from build123d import *

# Parameters (mm, degrees)
SKETCH1_R           = 4.75
BOSS_EXTRUDE1_DEPTH = 9
SKETCH2_R           = 7.5
BOSS_EXTRUDE2_DEPTH = 200
CUT_EXTRUDE1_START  = 4
SKETCH3_W           = 10
SKETCH3_H           = 10
CUT_EXTRUDE1_DEPTH  = 206.268965688
CIRPATTERN2_COUNT   = 3


with BuildPart() as part:
    # Sketch1 → Boss-Extrude1 (new body)
    with BuildSketch(Plane(origin=(0, 0, 0), x_dir=(1, 0, 0), z_dir=(0, 1, 0))):
        with Locations(Location((0, 0, 0), (0, 0, 270))):
            Circle(SKETCH1_R)
    extrude(amount=BOSS_EXTRUDE1_DEPTH)

    # Sketch2 → Boss-Extrude2 (add)
    with BuildSketch(Plane(origin=(0, 9, 0), x_dir=(1, 0, 0), z_dir=(0, 1, 0))):
        with Locations(Location((0, 0, 0), (0, 0, 270))):
            Circle(SKETCH2_R)
    extrude(amount=BOSS_EXTRUDE2_DEPTH)

    # Sketch3 → Cut-Extrude1 (cut, through all)
    with BuildSketch(Plane(origin=(0, 0, 0), x_dir=(0, 0, -1), z_dir=(1, 0, 0)).offset(CUT_EXTRUDE1_START)):
        with Locations((0, 204)):
            Rectangle(SKETCH3_W, SKETCH3_H)
    cut_extrude1 = extrude(amount=CUT_EXTRUDE1_DEPTH, mode=Mode.SUBTRACT)

    # CirPattern2: Cut-Extrude1 ×3 about axis
    cirpattern2_axis = Axis((0, 0, 0), (0, 1, 0))
    for i in range(1, CIRPATTERN2_COUNT):
        add(cut_extrude1.rotate(cirpattern2_axis, i * 360 / CIRPATTERN2_COUNT), mode=Mode.SUBTRACT)


solid = part.part
Input: part model. Units: mm. Frame: model coordinates. A direction names the side the tool comes from. Coordinates: 2 decimals unless noted, no trailing zeros. Order: outer loops, then holes, each group sorted by start corner. A loop starts at its lowest first (then second) coordinate and runs counter-clockwise, first axis right, second up. Notation, with made-up numbers: M 77,37 L 116,37 A23 cw 116,73 Z; hole C 78,-37 d3. An arc over 180 degrees is marked long. Write item = value, one per line. Start each with the question number.
(1) Section A-A on y = 189. Output: boundary loops of the cut face in (x, z), and give its area (3 significant figures).
(2) Pull-direction query (X, two-part tool) for faces 4 (the flat face through (5, 199, 0)), 5 (the flat face through (-1.94, 204.07, -3.5)), 6 (the cylindrical face through (0.33, 107.6, -7.493)); classes: released by +X, released by -X, zero draft, split by the parting line, or undercut.
(3) First-contact query: P1, Ø0.5, axis at x = 5, y = 202.5, coming from the +Z side; P2, Ø3.5, axis at x = -2.5, z = -3.5, coming from the +Y side; P3, Ø4, axis at x = -4.5, y = 144.5, coming from the -Z side; P4, Ø2, axis at y = 34, z = 4, coming from the -X side. Flat tips, straight axial feed; report the tip coordinate or a pass-through.
(4) Line query: line 1 along Y through (x, z) = (-2.5, 5.75); line 2 along Z through (x, y) = (0.25, 39.5); line 3 along X through (y, z) = (87, -4.5). Output: solid intervals per line, ascending. Write a range as [from, to].
(5) Reachability of faces 1 (the flat face through (4, 204, 0)), 2 (the flat face through (1, 209, 0)), 3 (the cylindrical face through (-2.89, 4.44, -3.77)) from +Z, -Z, +X, -X, +Y, -Y: full face, straight path, thin tool, end or side. Return the list, or none.
Result set:
q1.outline = C 0,0 d15
q1.area = 177 mm²
q2.face_4 = zero draft
q2.face_5 = undercut
q2.face_6 = split by the parting line
q3.P1 = 5.8
q3.P2 = 209
q3.P3 = -7.07
q3.P4 = -6.87
q4.line_1 = [9, 199]
q4.line_2 = [-7.5, 7.5]
q4.line_3 = [-6, 6]
q5.face_1 = +X, +Y
q5.face_2 = +Z, -Z, +X, -X, +Y
q5.face_3 = -Y
